Could you check a few things on this model? Use its own coordinates, in mm. A direction names the side the tool comes from. Round coordinates to 2 decimals unless told otherwise and drop trailing zeros. Write each question's results on one line, items separated by ' | '. Start each with the question number.
(1) Please list where these lines run through material, in increasing order: line 1 (Z direction, x = 5.75, y = 9.5); line 2 (Y direction, x = 1.25, z = -47); line 3 (Y direction, x = 2.5, z = -1.5). Write a range as [from, to].
(2) For P1, Ø0.8, axis at x = 3, y = 25, coming from the +Z side; P2, Ø0.5, axis at x = 1.5, y = 25, coming from the -Z side; P3, Ø2.5, axis at y = 9.525, z = -3.175, coming from the -X side; P4, Ø4.5, axis at y = 17.46, z = -47.62, coming from the -X side, each with a flat end and sliding along its axis, tell me the tip position at first contact or that it passes through.
(3) Imagine slicing it at A-A on x = 4.75. State how many separate pieces and enclosed holes the cut face has, then the cut area to 3 significant figures.
(4) Thinking about a two-plate mould opening in Z: for faces 5 (the cylindrical face through (3.9, 9.61, -45.73)), 6 (the flat face through (3, 13, 0)), 7 (the flat face through (6.35, 13, -25)), which applies, +Z half, -Z half, draft (parallel to the pull), parting line (faces both ways), or undercut?
(5) On a 3-axis mill with a long thin cutter (end or side, diameter ignored), from which of +Z, -Z, +X, -X, +Y, -Y can I reach the whole of each face in a straight line? I mean faces 1 (the flat face through (3, 25, -6.35)), 2 (the flat face through (3, 1, -44.45)), 3 (the flat face through (3, 1.588, -3)), 4 (the flat face through (3, 23.812, -48)). Say none if no direction works.
```python
from build123d import *

# Parameters (mm, degrees)
BOSS_EXTRUDE1_DEPTH                               = 6.35
CSK_FOR_6_FLAT_HEAD_MACHINE_SCREW_100_D           = 3.7973
CSK_FOR_6_FLAT_HEAD_MACHINE_SCREW_100_CSINK_D     = 7.0866
CSK_FOR_6_FLAT_HEAD_MACHINE_SCREW_100_CSINK_ANGLE = 100


with BuildPart() as part:
    # Sketch1 → Boss-Extrude1 (new body)
    with BuildSketch(Plane(origin=(0, 0, 0), x_dir=(0, 0, -1), z_dir=(1, 0, 0))):
        Polygon((44.45, 25.4), (25.4, 25.4), (25.4, 0), (44.45, 0), (44.45, 1.5875), (50.8, 1.5875), (50.8, 23.8125), (44.45, 23.8125), align=None)
        Polygon((25.4, 0), (25.4, 25.4), (6.35, 25.4), (6.35, 23.8125), (0, 23.8125), (0, 1.5875), (6.35, 1.5875), (6.35, 0), align=None)
    extrude(amount=BOSS_EXTRUDE1_DEPTH)

    # CSK for _6 Flat Head Machine Screw _100 (through all)
    with Locations(Plane.ZY):
        with Locations((-47.625, 17.4625), (-47.625, 9.525), (-3.175, 17.4625), (-3.175, 9.525)):
            CounterSinkHole(CSK_FOR_6_FLAT_HEAD_MACHINE_SCREW_100_D / 2, CSK_FOR_6_FLAT_HEAD_MACHINE_SCREW_100_CSINK_D / 2, counter_sink_angle=CSK_FOR_6_FLAT_HEAD_MACHINE_SCREW_100_CSINK_ANGLE)


solid = part.part
```
Response:
1) line 1: [-50.8, -49.52], [-45.73, -5.07], [-1.28, 0] | line 2: [1.59, 7.57], [11.48, 15.51], [19.42, 23.81] | line 3: [1.59, 8.63], [10.42, 16.57], [18.36, 23.81]
2) P1: z = -6.35 | P2: z = -44.45 | P3: through | P4: x = 1.08
3) separate pieces: 1 | enclosed holes: 4 | area: 1,200 mm²
4) face 5: undercut | face 6: +Z half | face 7: draft
5) face 1: +Z, +X, -X, +Y | face 2: -Z, +X, -X, -Y | face 3: +Z, +X, -X, -Y | face 4: -Z, +X, -X, +Y
